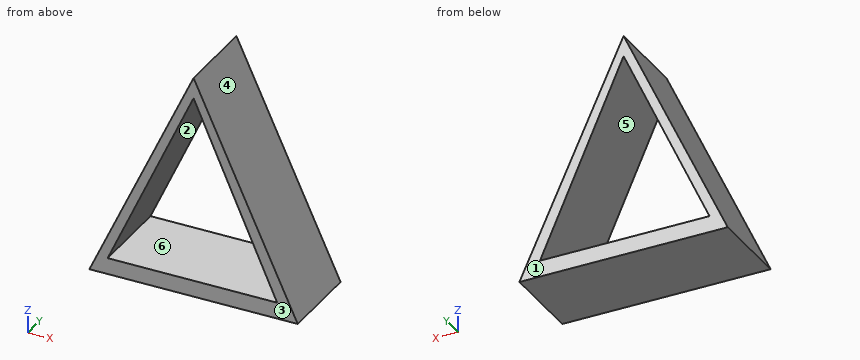
from build123d import *

# Parameters (mm, degrees)
F1_DEPTH = 25.4
F3_DEPTH = 50.8


with BuildPart() as f1:
    # F0 (on Front) → F1 (new body)
    with BuildSketch(Plane.XZ):
        Polygon((31.980053, -29.687206), (0, 39.477208), (-31.980053, -29.687206), align=None)
    extrude(amount=F1_DEPTH)

    # F2 (on Front) → F3 (cut)
    with BuildSketch(Plane.XZ):
        Polygon((25.663907, -24.663087), (0, 33.098578), (-26.37878, -24.663087), align=None)
    extrude(amount=F3_DEPTH, mode=Mode.SUBTRACT)


solid = f1.part
Could you check a few things on this model? Use its own coordinates, in mm. Face numbers are marked on the shaded views. A direction names the side the tool comes from. Give positions to 0.01 mm unless a question says otherwise; leave off trailing zeros. Order: outer loops, then holes, each group sorted by start corner. A loop starts at its lowest first (then second) coordinate and runs counter-clockwise, first axis right, second up.
1. Suppose I cut it at A-A (z = 30.5). List the corners of the cut face in (x, y) for me, plus the area to 3 significant figures.
2. Suppose I cut it at B-B (y = -12.25). List the corners of the cut face in (x, z) for me, plus the area to 3 significant figures.
3. Suppose I cut it at C-C (x = -5.5). List the corners of the cut face in (y, z) for me, plus the area to 3 significant figures.
4. We'd pull the mould along X, two halves only. Please class the marked faces 3, 4, 5 and 6: pulls with the +X half, pulls with the -X half, needs draft (parallel to the pull), parting line crosses it, or undercut.
5. I need wall thicknesses on L1, parallel to Z at x = -0.5, y = -4; L2, parallel to Z at x = -2.5, y = -19.75; L3, parallel to X at y = -7.75, z = -9. Which ranges of each line are inside material? Lowest first, please.
6. Will these pins go through, and if not, where does the flat tip stop? P1, Ø7.5, axis at x = -7, y = -18, coming from the +Z side; P2, Ø12, axis at x = -12, z = -3.5, coming from the -Y side; P3, Ø8, axis at y = -4, z = 9, coming from the +X side; P4, Ø3, axis at x = 5.5, y = -22.5, coming from the +Z side.
7. For the marked faces 1 and 2, which set-ups out of +Z, -Z, +X, -X, +Y, -Y let a thin tool reach every point of the face, with its end or its side?
8. Suppose I cut it at D-D (x = 26.5). List the corners of the cut face in (y, z) for me, plus the area to 3 significant figures.
Solved:
1. outline: (-4.15, -25.4) - (-1.19, -25.4) - (-1.19, 0) - (-4.15, 0) - close; (1.15, -25.4) - (4.15, -25.4) - (4.15, 0) - (1.15, 0) - close
1. area: 151 mm2
2. outline: (-31.98, -29.69) - (31.98, -29.69) - (0, 39.48) - close; hole (-26.38, -24.66) - (25.66, -24.66) - (0, 33.1) - close
2. area: 709 mm2
3. outline: (-25.4, -29.69) - (0, -29.69) - (0, -24.66) - (-25.4, -24.66) - close; (-25.4, 21.06) - (0, 21.06) - (0, 27.58) - (-25.4, 27.58) - close
3. area: 293 mm2
4. face 3: needs draft
4. face 4: pulls with the +X half
4. face 5: undercut
4. face 6: undercut
5. L1: z = -29.69 to -24.66, 32 to 38.4
5. L2: z = -29.69 to -24.66, 27.62 to 34.07
5. L3: x = -22.41 to -19.23, 18.7 to 22.41
6. P1: stops at z = 32.45
6. P2: stops at y = -25.4
6. P3: stops at x = 15.94
6. P4: stops at z = 30.83
7. face 1: +Z, -Z, +X, -X, +Y
7. face 2: +Y, -Y
8. outline: (-25.4, -29.69) - (0, -29.69) - (0, -17.84) - (-25.4, -17.84) - close
8. area: 301 mm2
